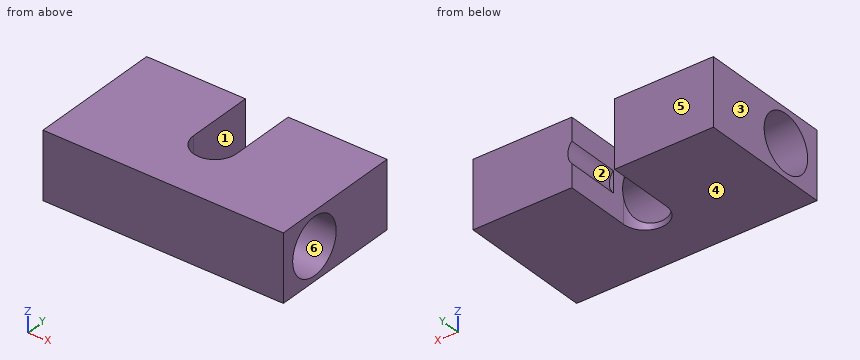
from build123d import *

# Parameters (mm, degrees)
F1_DEPTH = 25
F2_R     = 10.5
F3_DEPTH = 90.001
F4_R     = 6
F5_DEPTH = 20


with BuildPart() as f1:
    # F0 (on Top) → F1 (new body)
    with BuildSketch(Plane.XY):
        with BuildLine():
            Line((0, 50), (0, 0))
            Line((0, 0), (90, 0))
            Line((90, 0), (90, 50))
            Line((90, 50), (53, 50))
            Line((53, 50), (53, 25))
            ThreePointArc((53, 25), (45, 17), (37, 25))
            Line((37, 25), (37, 50))
            Line((37, 50), (0, 50))
        make_face()
    extrude(amount=F1_DEPTH)

    # F2 (on face) → F3 (cut, through all)
    with BuildSketch(Plane(origin=(0, 0, 0), x_dir=(0, -1, 0), z_dir=(-1, 0, 0))):
        with Locations((-15, 12.5)):
            Circle(F2_R)
    extrude(amount=-F3_DEPTH, mode=Mode.SUBTRACT)

    # F4 (on face) → F5 (cut)
    with BuildSketch(Plane(origin=(0, 50, 0), x_dir=(-1, 0, 0), z_dir=(0, 1, 0))):
        with Locations((-48.5, 12.5)):
            Circle(F4_R)
        with Locations((11.5, 12.5)):
            Circle(F4_R)
    extrude(amount=-F5_DEPTH, mode=Mode.SUBTRACT)


solid = f1.part
Could you check a few things on this model? Use its own coordinates, in mm. Face numbers are marked on the shaded views. A direction names the side the tool comes from. Give positions to 0.01 mm unless a question says otherwise; leave off trailing zeros. Order: outer loops, then holes, each group sorted by start corner. A loop starts at its lowest first (then second) coordinate and runs counter-clockwise, first axis right, second up. Notation, with made-up numbers: (-38, -36.75) - (1, -36.75) arc R15 cw to (1, -8.75) - close; hole circle Ø3 at (39, 62). An arc over 180 degrees is marked (long way). One line per question, with ' | ' between items. Start each with the question number.
Item 1: Thinking about a two-plate mould opening in Z: for the marked faces 4, 5 and 6, which applies, pulls with the +Z half, pulls with the -Z half, needs draft (parallel to the pull), parting line crosses it, or undercut?
Item 2: For the marked faces 1, 2 and 3, which set-ups out of +Z, -Z, +X, -X, +Y, -Y let a thin tool reach every point of the face, with its end or its side?
Item 3: I'm going to push flat-ended pins straight in: pin 1 Ø6 at (y, z) = (13.5, 18) entering from -X; pin 2 Ø1.6 at (x, z) = (53.5, 12.5) entering from +Y. Where does each tip first touch, or does it pass through?
Item 4: I want a section at D-D on y = 15. Write out the boundary of the cut face in (x, z).
Item 5: I want a section at C-C on x = 25.5. Write out the boundary of the cut face in (y, z), then the cut area to 3 significant figures.
Item 6: I want a section at A-A on y = 27. Write out the boundary of the cut face in (x, z), then the cut area to 3 significant figures.
Item 7: I need wall thicknesses on probe 1 along Z at (x, y) = (66, 15); probe 2 along Y at (x, z) = (35, 12.5); probe 3 along X at (y, z) = (42.5, 21). Which ranges of each line are inside material? Lowest first, please. Write a range as [from, to].
Item 8: I want a section at B-B on z = 12.5. Write out the boundary of the cut face in (x, y).
Verdict:
1) face 4: pulls with the -Z half | face 5: needs draft | face 6: undercut
2) face 1: +Z, -Z, +Y | face 2: +Y | face 3: +Z, -Z, -X, +Y, -Y
3) pin 1: through | pin 2: y = 30
4) outline: (0, 0) - (90, 0) - (90, 2) - (0, 2) - close; (0, 23) - (90, 23) - (90, 25) - (0, 25) - close
5) outline: (0, 0) - (50, 0) - (50, 25) - (0, 25) - close; hole circle Ø21 at (15, 12.5) | area: 904 mm^2
6) outline: (0, 0) - (37, 0) - (37, 25) - (0, 25) - close; (53, 0) - (90, 0) - (90, 25) - (53, 25) - close | area: 1,850 mm^2
7) probe 1: [0, 2], [23, 25] | probe 2: [0, 4.5], [25.5, 50] | probe 3: [0, 37], [53, 90]
8) outline: (0, 0) - (90, 0) - (90, 4.5) - (0, 4.5) - close; (0, 25.5) - (37, 25.5) - (37, 50) - (0, 50) - close; (53, 25.5) - (90, 25.5) - (90, 50) - (54.5, 50) - (54.5, 30) - (53, 30) - close
